Design review of the part built by this model. Coordinates are the model's own, in mm. A direction names the side the tool comes from. Give positions to 0.01 mm unless a question says otherwise; leave off trailing zeros.
Autodesk Inventor part; units mm, degrees
ref_plane "YZ Plane" through (0, 0, 0) normal (1, 0, 0) x (0, 1, 0)
ref_plane "XZ Plane" through (0, 0, 0) normal (0, 1, 0) x (-1, 0, 0)
ref_plane "XY Plane" through (0, 0, 0) normal (0, 0, 1) x (1, 0, 0)
sketch "Sketch1" plane through (0, 0, 0) normal (0, 1, 0) x (-1, 0, 0)
  line L0 (31.75, 74.8157) -> (-31.75, 74.8157)
  line L1 (-31.75, 74.8157) -> (-31.75, -74.8157)
  line L2 (-31.75, -74.8157) -> (31.75, -74.8157)
  line L3 (31.75, -74.8157) -> (31.75, 74.8157)
  line L4 (0, 0) -> (31.75, 0) construction
  line L5 (0, 0) -> (0, 74.8157) construction
  line L6 (0, 0) -> (-31.75, 0) construction
  line L7 (0, 0) -> (0, -74.8157) construction
  dimension "d0" = 63.5
  dimension "d1" = 149.6314
extrude "Extrusion1" add sketch "Sketch1" along normal blind 110.8075
sketch "Sketch2" plane through (0, 110.8075, 0) normal (0, 1, 0) x (1, 0, 0)
  line L0 (-31.75, -74.8157) -> (31.75, -74.8157)
  line L1 (31.75, -74.8157) -> (31.75, 74.8157)
  line L2 (31.75, 74.8157) -> (-31.75, 74.8157)
  line L3 (-31.75, 74.8157) -> (-31.75, -74.8157)
  line L4 (-30.1498, -73.2155) -> (30.1498, -73.2155)
  line L5 (30.1498, -73.2155) -> (30.1498, 73.2155)
  line L6 (30.1498, 73.2155) -> (-30.1498, 73.2155)
  line L7 (-30.1498, 73.2155) -> (-30.1498, -73.2155)
  point P0 (0, 0)
  dimension "d4" = 1.6002
extrude "Extrusion2" cut sketch "Sketch2" against normal blind 7.4422
sketch "Sketch3" plane through (0, 103.3653, 0) normal (0, 1, 0) x (1, 0, 0)
  line L0 (-30.1498, 73.2155) -> (-30.1498, 53.2257)
  line L1 (30.1498, 73.2155) -> (-30.1498, 73.2155)
  line L2 (31.75, 74.8157) -> (31.75, 53.2257)
  line L3 (-31.75, 74.8157) -> (31.75, 74.8157)
  line L4 (30.1498, 73.2155) -> (-30.1498, 73.2155)
  line L5 (-31.75, 53.2257) -> (-30.1498, 53.2257)
  line L6 (31.75, 53.2257) -> (30.1498, 53.2257)
  line L7 (30.1498, 53.2257) -> (30.1498, 73.2155)
  line L8 (-31.75, 53.2257) -> (-31.75, 74.8157)
  point P0 (0, 0)
  dimension "d7" = 21.59
sketch "Sketch4" plane through (0, 103.3653, 0) normal (0, 1, 0) x (1, 0, 0)
  line L0 (-31.75, 74.8157) -> (31.75, 74.8157)
  line L1 (30.1498, 73.2155) -> (-30.1498, 73.2155)
  line L2 (-31.75, 74.8157) -> (-31.75, 53.2257)
  line L3 (-31.75, 53.2257) -> (-30.1498, 53.2257)
  line L4 (-30.1498, 73.2155) -> (-30.1498, 53.2257)
  line L5 (0, 73.2155) -> (0, 74.8157) construction
  line L6 (31.75, 74.8157) -> (31.75, 53.2257)
  line L7 (31.75, 53.2257) -> (30.1498, 53.2257)
  line L8 (30.1498, 73.2155) -> (30.1498, 53.2257)
  point P0 (0, 0)
  dimension "d8" = 21.59
extrude "Extrusion3" add sketch "Sketch4" along normal up to surface (7.4422 mm away)
sketch "Sketch5" plane through (-31.75, 0, 74.8157) normal (0, 0, 1) x (1, 0, 0)
  line L0 (22.0103, 51.8449) -> (31.9769, 51.8449) construction
  line L1 (31.9769, 51.8449) -> (31.9769, 48.6882) construction
  line L2 (31.9769, 48.6882) -> (22.0103, 48.6882) construction
  line L3 (22.0103, 48.6882) -> (22.0103, 51.8449) construction
sketch "Sketch6" plane through (31.75, 0, -74.8157) normal (0, 0, -1) x (-1, 0, 0)
  line L0 (18.5743, 56.7919) -> (44.5786, 56.7919) construction
  line L1 (44.5786, 56.7919) -> (44.5786, 50.439) construction
  line L2 (44.5786, 50.439) -> (18.5743, 50.439) construction
  line L3 (18.5743, 50.439) -> (18.5743, 56.7919) construction
sketch "Sketch7" plane through (0, 110.8075, 0) normal (0, 1, 0) x (1, 0, 0)
  line L0 (27.94, 71.0057) -> (13.97, 71.0057)
  line L1 (13.97, 71.0057) -> (13.97, 57.0357)
  line L2 (13.97, 57.0357) -> (27.94, 57.0357)
  line L3 (27.94, 57.0357) -> (27.94, 71.0057)
  line L4 (31.75, 74.8157) -> (31.75, 53.2257) construction
  line L5 (-31.75, 74.8157) -> (31.75, 74.8157) construction
  line L6 (0, 74.8157) -> (0, -73.2155) construction
  line L7 (-30.1498, -73.2155) -> (30.1498, -73.2155) construction
  line L8 (-27.94, 71.0057) -> (-13.97, 71.0057)
  line L9 (-13.97, 71.0057) -> (-13.97, 57.0357)
  line L10 (-13.97, 57.0357) -> (-27.94, 57.0357)
  line L11 (-27.94, 57.0357) -> (-27.94, 71.0057)
  point P0 (0, 0)
  dimension "d11" = 13.97
  dimension "d12" = 3.81
  dimension "d13" = 3.81
extrude "Extrusion4" add sketch "Sketch7" along normal blind 0.254
equation "\"d13\" = d12"
properties part number "BotBattery"
(1) To check wall thickness, follow L1, parallel to Y at x = -9, z = -20; L2, parallel to X at y = 105, z = 35.5. State the ranges of each line that lie inside material, in increasing order.
Resolved:
L1: y = 0 to 110.81
L2: x = -30.15 to 30.15
(2) Tool access review of faces 1 (the face through (0, 0, 1)), 2 (the face through (-30.15, 107, 9)), 3 (the face through (31.75, 55, -1)), 4 (the face through (30.15, 107, 11)), 5 (the face through (0, 107, 73.216)): name each direction out of +Z, -Z, +X, -X, +Y, -Y from which nothing blocks a thin tool from reaching the whole face with its end or side.
Resolved:
face 1: +Z, -Z, +X, -X, -Y
face 2: +Z, -X, +Y
face 3: +Z, -Z, +X, +Y, -Y
face 4: +Z, +X, +Y
face 5: +Z, +X, -X, +Y
(3) Clearance check with flat-ended pins moving along their axes: P1, Ø6, axis at y = 107, z = 34.5, coming from the -X side; P2, Ø19, axis at x = -5.5, z = 35, coming from the +Y side; P3, Ø0.8, axis at x = -31, y = 106, coming from the +Z side. State where each tip first meets the part, or that it passes through.
Resolved:
P1: stops at x = -30.15
P2: stops at y = 110.81
P3: stops at z = -53.23
